Check sheet for the drawn part. Datum: minimum x, y, z corner. Units: mm. A direction names the side the tool comes from. Round coordinates to 2 decimals unless told otherwise and drop trailing zeros. Loops run counter-clockwise (first coordinate to the right, second up) from the corner with the lowest first, then second, coordinate; pieces in that order, holes last. Notation, with made-up numbers: (-20.5, -27) - (-9.5, -27) arc R16 cw to (-9.5, -23) - close; hole circle Ø11 at (-22.5, -2). An arc over 180 degrees is marked (long way). Use CSV: the item, a comma, the result in double quotes.
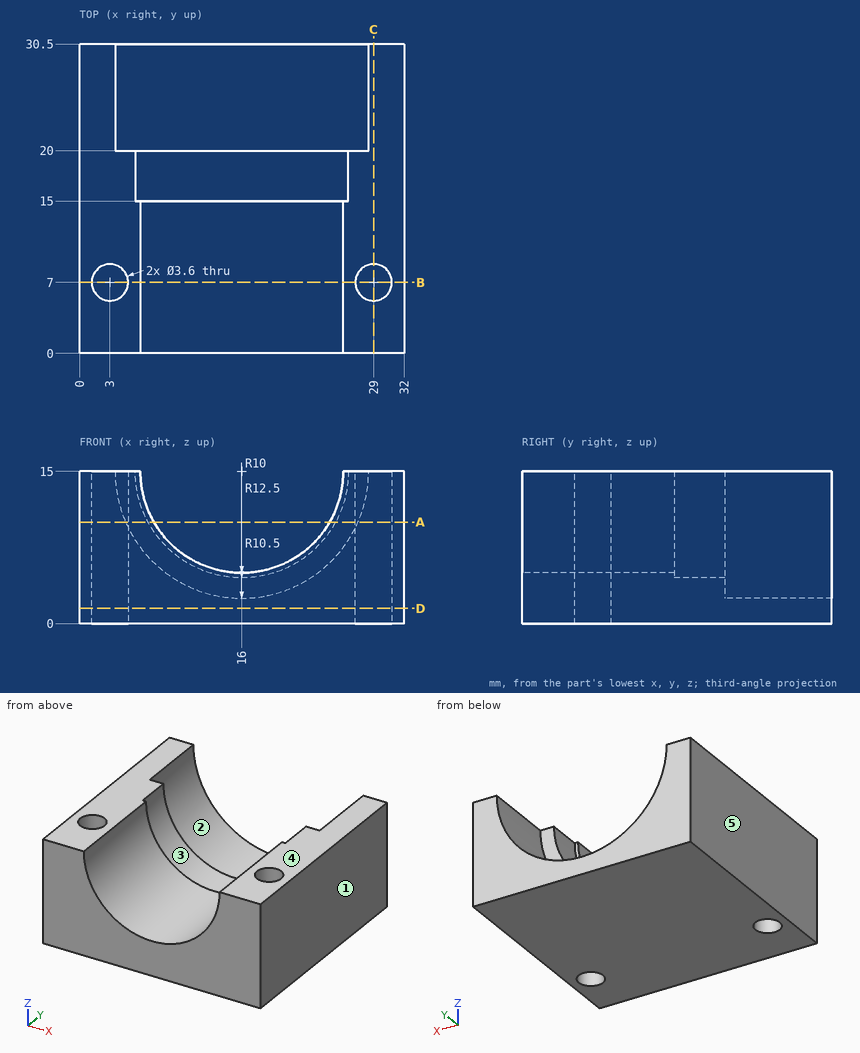
1) Cross-section at C-C, the plane x = 29. Record the cut outline in (y, z), then the cut area to 4 significant figures.
Returned:
outline,"(0, 0) - (5.2, 0) - (5.2, 15) - (0, 15) - close; (8.8, 0) - (30.5, 0) - (30.5, 15) - (8.8, 15) - close"
area,"403.5 mm²"
2) Access from +Z, -Z, +X, -X, +Y, -Y to the whole of each face (thin tool, end or side, straight path). Record for the marked faces 1 and 2.
Returned:
face 1,"+Z, -Z, +X, +Y, -Y"
face 2,"+Z, +Y"
3) Gauge pin test, flat ends, axial feed: pin 1 Ø2 at (x, y) = (19.5, 27) entering from +Z; pin 2 Ø1 at (y, z) = (17, 6) entering from -X; pin 3 Ø3 at (x, y) = (3, 7) entering from +Z. Record the tip position at first contact, or that the pin passes through.
Returned:
pin 1,"stops at z = 3.34"
pin 2,"stops at x = 0"
pin 3,"passes through"
4) Cross-section at D-D, the plane z = 1.5. Record the cut outline in (x, y).
Returned:
outline,"(0, 0) - (32, 0) - (32, 30.5) - (0, 30.5) - close; hole circle Ø3.6 at (3, 7); hole circle Ø3.6 at (29, 7)"
5) Cross-section at A-A, the plane z = 10. Record the cut outline in (x, y), then the cut area to 3 significant figures.
Returned:
outline,"(0, 0) - (7.34, 0) - (7.34, 15) - (6.77, 15) - (6.77, 20) - (4.54, 20) - (4.54, 30.5) - (0, 30.5) - close; (24.66, 0) - (32, 0) - (32, 30.5) - (27.46, 30.5) - (27.46, 20) - (25.23, 20) - (25.23, 15) - (24.66, 15) - close; hole circle Ø3.6 at (3, 7); hole circle Ø3.6 at (29, 7)"
area,"363 mm²"
6) Mould release check, pull along X, two halves, no side actions. Record for the marked faces 3, 4 and 5: +X half, -X half, draft (parallel to the pull), parting line (faces both ways), or undercut.
Returned:
face 3,"undercut"
face 4,"draft"
face 5,"-X half"
7) Cross-section at B-B, the plane y = 7. Record the cut outline in (x, z).
Returned:
outline,"(0, 0) - (1.2, 0) - (1.2, 15) - (0, 15) - close; (4.8, 0) - (27.2, 0) - (27.2, 15) - (26, 15) arc R10 cw to (6, 15) - (4.8, 15) - close; (30.8, 0) - (32, 0) - (32, 15) - (30.8, 15) - close"
8) Thickness scan on probe 1 along Y at (x, z) = (3, 7.75); probe 2 along X at (y, z) = (5.5, 11.5); probe 3 along X at (y, z) = (2.5, 14.75). Record the ranges inside material, lowest first. Write a range as [from, to].
Returned:
probe 1,"y = [0, 5.2], [8.8, 30.5]"
probe 2,"x = [0, 2.01], [3.99, 6.63], [25.37, 28.01], [29.99, 32]"
probe 3,"x = [0, 6], [26, 32]"
